Autodesk Inventor part; units mm, degrees
ref_plane "YZ Plane" through (0, 0, 0) normal (1, 0, 0) x (0, 1, 0)
ref_plane "XZ Plane" through (0, 0, 0) normal (0, 1, 0) x (-1, 0, 0)
ref_plane "XY Plane" through (0, 0, 0) normal (0, 0, 1) x (1, 0, 0)
sketch "Sketch1" plane through (0, 0, 0) normal (0, 1, 0) x (-1, 0, 0)
  line L0 (-16, 16) -> (-16, -16)
  line L1 (-16, -16) -> (16, -16)
  line L2 (16, -16) -> (16, 16)
  line L3 (16, 16) -> (-16, 16)
  line L4 (-16, 16) -> (16, -16) construction
  line L5 (-16, -16) -> (16, 16) construction
  point P0 (0, 0)
  dimension "d0" = 32
  dimension "d1" = 32
extrude "Extrusion1" add sketch "Sketch1" along normal blind 1.6
sketch "Sketch2" plane through (0, 1.6, 0) normal (0, 1, 0) x (1, 0, 0)
  line L0 (-8, -8) -> (-8, 8)
  line L1 (-8, 8) -> (8, 8)
  line L2 (8, 8) -> (8, -8)
  line L3 (8, -8) -> (-8, -8)
  line L4 (-8, -8) -> (8, 8) construction
  line L5 (-8, 8) -> (8, -8) construction
  point P0 (0, 0)
  dimension "d4" = 16
  dimension "d5" = 16
extrude "Extrusion2" add sketch "Sketch2" along normal blind 6
sketch "Sketch3" plane through (0, 7.6, 0) normal (0, 1, 0) x (1, 0, 0)
  circle A0 centre (0, 0) radius 7.5
  dimension "d8" = 15
extrude "Extrusion3" add sketch "Sketch3" along normal blind 10
sketch "Sketch4" plane through (0, 1.6, 0) normal (0, 1, 0) x (1, 0, 0)
  line L0 (-13.75, -13.75) -> (-13.75, 13.75)
  line L1 (-13.75, 13.75) -> (13.75, 13.75)
  line L2 (13.75, 13.75) -> (13.75, -13.75)
  line L3 (13.75, -13.75) -> (-13.75, -13.75)
  line L4 (-13.75, -13.75) -> (13.75, 13.75) construction
  line L5 (-13.75, 13.75) -> (13.75, -13.75) construction
  point P0 (0, 0)
  dimension "d11" = 27.5
  dimension "d12" = 27.5
hole "Hole1" at (-13.75, 1.6, 13.75) at (13.75, 1.6, 13.75) at (13.75, 1.6, -13.75) at (-13.75, 1.6, -13.75) direction (0, -1, 0) diameter 2 depth 7
properties part number "cam_1"
Model file for the job. Use its own axes, mm. A direction names the side the tool comes from. Give positions to 0.01 mm unless a question says otherwise; leave off trailing zeros. Order: outer loops, then holes, each group sorted by start corner. A loop starts at its lowest first (then second) coordinate and runs counter-clockwise, first axis right, second up. Notation, with made-up numbers: (-10, 33) - (42, 33) arc R24 ccw to (42, 46) - close; hole circle Ø8 at (71, -23). An arc over 180 degrees is marked (long way). Write item = value, one per line. Start each with the question number.
1. Cut at A-A, the plane z = 13.75. List the corners of the cut face in (x, y).
2. Which spindle directions (+Z, -Z, +X, -X, +Y, -Y) get a long thin tool onto all of the face, cutting with end or side? Do faces 4 (the cylindrical face through (-7.493, 12.53, 0.33)), 5 (the flat face through (0, 5, -8)), 6 (the flat face through (8, 5, 0)). Say none if no direction does.
3. Cut at B-B, the plane x = 13.75. List the corners of the cut face in (y, z).
4. Cut at C-C, the plane z = 0. List the corners of the cut face in (x, y).
5. Probe line 1 along X through (y, z) = (0.4, 13.75); line 2 along Z through (x, y) = (-2.5, 4.5). List the from-to ranges inside material, lowest first.
6. Two-plate mould, pull along X, no slides. Class faces 1 (the flat face through (-8, 5, 0)), 2 (the cylindrical face through (14.64, 0.79, -13.29)), 3 (the flat face through (0, 1, -16)): pulls with the +X half, pulls with the -X half, needs draft (parallel to the pull), parting line crosses it, or undercut.
7. Drop flat-ended pins along their axis: P1, Ø5, axis at x = 2, y = 5, coming from the +Z side; P2, Ø1.5, axis at x = -1.5, z = -12.5, coming from the +Y side; P3, Ø2, axis at x = 7.5, y = 13, coming from the +Z side. Give the stop position or say it passes through.
8. Cut at D-D, the plane x = -5. List the corners of the cut face in (y, z).
Taken from the geometry:
q1.outline = (-16, 0) - (-14.75, 0) - (-14.75, 1.6) - (-16, 1.6) - close; (-12.75, 0) - (12.75, 0) - (12.75, 1.6) - (-12.75, 1.6) - close; (14.75, 0) - (16, 0) - (16, 1.6) - (14.75, 1.6) - close
q2.face_4 = +Y
q2.face_5 = -Z, +X, -X, +Y
q2.face_6 = +Z, -Z, +X, +Y
q3.outline = (0, -16) - (1.6, -16) - (1.6, -14.75) - (0, -14.75) - close; (0, -12.75) - (1.6, -12.75) - (1.6, 12.75) - (0, 12.75) - close; (0, 14.75) - (1.6, 14.75) - (1.6, 16) - (0, 16) - close
q4.outline = (-16, 0) - (16, 0) - (16, 1.6) - (8, 1.6) - (8, 7.6) - (7.5, 7.6) - (7.5, 17.6) - (-7.5, 17.6) - (-7.5, 7.6) - (-8, 7.6) - (-8, 1.6) - (-16, 1.6) - close
q5.line_1 = -16 to -14.75, -12.75 to 12.75, 14.75 to 16
q5.line_2 = -8 to 8
q6.face_1 = pulls with the -X half
q6.face_2 = undercut
q6.face_3 = needs draft
q7.P1 = 8
q7.P2 = 1.6
q7.P3 = 3.74
q8.outline = (0, -16) - (1.6, -16) - (1.6, -8) - (7.6, -8) - (7.6, -5.59) - (17.6, -5.59) - (17.6, 5.59) - (7.6, 5.59) - (7.6, 8) - (1.6, 8) - (1.6, 16) - (0, 16) - close
